Part model, mm, in its own coordinate system. Face numbers are marked on the shaded views. Round coordinates to 2 decimals unless told otherwise and drop trailing zeros. Loops run counter-clockwise (first coordinate to the right, second up) from the corner with the lowest first, then second, coordinate; pieces in that order, holes last. Notation, with made-up numbers: M 22.5,28.25 L 55.5,28.25 A19 cw 55.5,62.25 Z; hole C 12.5,44 d4. An arc over 180 degrees is marked long. Put each result on its own line as item: value. Start each with the question number.
1) Slice it at C-C on z = -52. Give the cut face in (x, y).
2) Drop flat-ended pins along their axis: pin 1 Ø3 at (x, z) = (-43, -28.5) entering from +Y; pin 2 Ø2 at (x, z) = (16.5, -47) entering from +Y; pin 3 Ø4 at (x, z) = (27.5, -28) entering from +Y. Give the stop position or say it passes through.
3) Probe line 1 along X through (y, z) = (0, -41); line 2 along Y through (x, z) = (4.5, -8.5). List the from-to ranges inside material, lowest first.
4) Slice it at A-A on x = 0. Give the cut face in (y, z), then the cut area to 3 significant figures.
5) Pull direction Y, two halves, no side cores. Call the marked faces 1, 2 and 3: +Y half, -Y half, draft (parallel to the pull), parting line (faces both ways), or undercut.
Autodesk Inventor part; units mm, degrees
ref_plane "YZ Plane" through (0, 0, 0) normal (1, 0, 0) x (0, 1, 0)
ref_plane "XZ Plane" through (0, 0, 0) normal (0, 1, 0) x (-1, 0, 0)
ref_plane "XY Plane" through (0, 0, 0) normal (0, 0, 1) x (1, 0, 0)
sketch "Sketch2" plane through (0, 0, 0) normal (1, 0, 0) x (0, 1, 0)
  line L0 (0, 0) -> (0, -57.2)
  line L1 (48.69, -57.2) -> (48.69, 0)
  line L2 (48.69, 0) -> (59.5, 0)
  line L3 (59.5, 0) -> (59.5, -2.29)
  line L4 (58.9736, -3.0418) -> (52.116, -5.5377)
  line L5 (50.8, -7.4171) -> (50.8, -57.2)
  line L6 (50.8, -57.2) -> (48.69, -57.2)
  arc A0 (58.9736, -3.0418) -> (59.5, -2.29) centre (58.7, -2.29) ccw
  arc A1 (52.116, -5.5377) -> (50.8, -7.4171) centre (52.8, -7.4171) ccw
  dimension "OD" = 101.6
  dimension "THW" = 2.11
  dimension "L" = 57.2
  dimension "d3" = 119
  dimension "d4" = 0.8
  dimension "d5" = 2.29
  dimension "d6" = 2
  dimension "d7" = 20
revolve "Revolution1" add sketch "Sketch2" angle 360 about axis through (0, 0, 0) along (0, 0, -1)
properties part number "Ferrule-101.6" material "Stainless Steel, 316L"
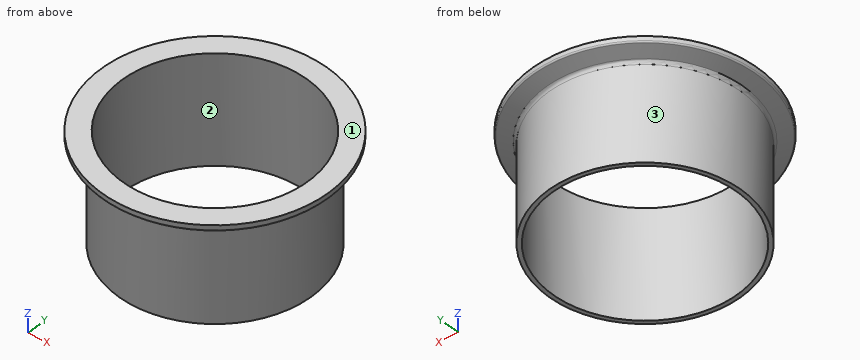
Recorded:
1. outline: C 0,0 d101.6; hole C 0,0 d97.38
2. pin 1: stops at y = 29.3
2. pin 2: stops at y = 48.38
2. pin 3: stops at y = 43.94
3. line 1: x = -50.8 to -48.69, 48.69 to 50.8
3. line 2: y = -50.6 to -48.48, 48.48 to 50.6
4. outline: M -59.5,-2.29 A0.8 ccw -58.97,-3.04 L -52.12,-5.54 A2 cw -50.8,-7.42 L -50.8,-57.2 L -48.69,-57.2 L -48.69,0 L -59.5,0 Z; M 48.69,-57.2 L 50.8,-57.2 L 50.8,-7.42 A2 cw 52.12,-5.54 L 58.97,-3.04 A0.8 ccw 59.5,-2.29 L 59.5,0 L 48.69,0 Z
4. area: 319 mm2
5. face 1: draft
5. face 2: undercut
5. face 3: parting line
